Verification items for the finished model (mm, model axes). Face numbers are marked on the shaded views. A direction names the side the tool comes from. Give positions to 0.01 mm unless a question says otherwise; leave off trailing zeros. Write each loop counter-clockwise with the first axis right and the second up, starting at its lowest first coordinate (ties: lowest second). Pieces come first, ordered by that corner, then holes. Notation, with made-up numbers: (16, 0.5) -> (57, 0.5) arc R27 ccw to (57, 31.5) -> close; hole circle Ø6 at (22, 4). An arc over 180 degrees is marked (long way). Write item = value, one per line.
from build123d import *

# Parameters (mm, degrees)
F0_R     = 3.175
F1_DEPTH = 23.8252
F3_DEPTH = 6.096
F5_DEPTH = 6.096
F6_SIZE  = 0.254


with BuildPart() as f1:
    # F0 (on Front) → F1 (new body)
    with BuildSketch(Plane.XZ):
        Circle(F0_R)
    extrude(amount=F1_DEPTH)

    # F2 (on face) → F3 (cut)
    with BuildSketch(Plane(origin=(0, 0, 0), x_dir=(-1, 0, 0), z_dir=(0, 1, 0))):
        with BuildLine():
            ThreePointArc((1.554181, 2.7686), (0, 3.175), (-1.554181, 2.7686))
            Line((-1.554181, 2.7686), (1.554181, 2.7686))
        make_face()
    extrude(amount=-F3_DEPTH, mode=Mode.SUBTRACT)

    # F4 (on face) → F5 (cut)
    with BuildSketch(Plane.XZ.offset(23.8252)):
        with BuildLine():
            ThreePointArc((1.554181, 2.7686), (0, 3.175), (-1.554181, 2.7686))
            Line((-1.554181, 2.7686), (1.554181, 2.7686))
        make_face()
    extrude(amount=-F5_DEPTH, mode=Mode.SUBTRACT)

    # F6
    f6_edges = [f1.edges().sort_by_distance(p)[0] for p in [
        (-1.604073, 0, -2.739995),
        (-1.604073, -23.8252, -2.739995),
    ]]
    chamfer(f6_edges, length=F6_SIZE)


solid = f1.part
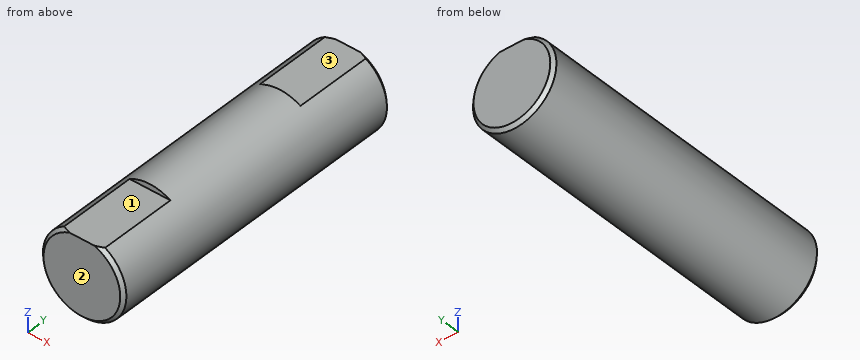
Item 1: Material ranges on line 1 (Z direction, x = -1.25, y = -15.5); line 2 (Z direction, x = -1, y = -12.25); line 3 (X direction, y = -18.25, z = -1.75), recorded low to high.
Response values:
line_1 = -2.92 to 2.92
line_2 = -3.01 to 3.01
line_3 = -2.65 to 2.65
Item 2: Sectioned sample at B-B on y = -4. Record the cut outline in (x, z) (3 decimals), then the cut area to 3 significant figures.
Response values:
outline = (-1.554, 2.769) arc R3.175 ccw (long way) to (1.554, 2.769) -> close
area = 30.8 mm^2
Item 3: Sectioned sample at C-C on y = -8. Record the cut outline in (x, z) (3 decimals).
Response values:
outline = circle Ø6.35 at (0, 0)
Item 4: Sectioned sample at A-A on x = 0. Record the cut outline in (y, z) (3 decimals).
Response values:
outline = (-23.825, -2.921) -> (-23.571, -3.175) -> (-0.254, -3.175) -> (0, -2.921) -> (0, 2.769) -> (-6.096, 2.769) -> (-6.096, 3.175) -> (-17.729, 3.175) -> (-17.729, 2.769) -> (-23.825, 2.769) -> close
Item 5: Go/stop test with flat-tipped pins: P1, Ø1, axis at y = -10, z = 1, coming from the +X side; P2, Ø1, axis at x = -2, y = -7.5, coming from the -Z side; P3, Ø1.5, axis at x = -1, y = -9.5, coming from the +Z side. Record where each tip stops, or that it passes through.
Response values:
P1 = 3.14
P2 = -2.8
P3 = 3.17
Item 6: Set-up check for the marked faces 1, 2 and 3: record each of +Z, -Z, +X, -X, +Y, -Y from which the full face is reachable in a straight line by a thin tool's end or side.
Response values:
face_1 = +Z, +X, -X, -Y
face_2 = +Z, -Z, +X, -X, -Y
face_3 = +Z, +X, -X, +Y
